```python
from build123d import *

# Parameters (mm, degrees)
SKETCH_1_W                     = 144
SKETCH_1_H                     = 144
SKETCH_1_R                     = 1.65
SKETCH_1_W_2                   = 11.212967435
SKETCH_1_H_2                   = 64.771297792
SKETCH_1_W_3                   = 88
SKETCH_1_H_3                   = 84
EXTRUDE_79X92_DEPTH            = 2
SKETCH_2_R                     = 2.75
M3_D5P5_1P1_90_DEPTH           = 1.1
M3_D5P5_1P1_90_DRAFT           = 45
M3_D5P5_1P1_90_PROFILE_2_DEPTH = 1.1
M3_D5P5_1P1_90_PROFILE_2_DRAFT = 45
M3_D5P5_1P1_90_PROFILE_3_DEPTH = 1.1
M3_D5P5_1P1_90_PROFILE_3_DRAFT = 45
M3_D5P5_1P1_90_PROFILE_4_DEPTH = 1.1
M3_D5P5_1P1_90_PROFILE_4_DRAFT = 45
CHAMFER_1_SIZE                 = 13


with BuildPart() as part:
    # 草图1 → 几何镂空托板_原装79x92孔距 (new body)
    with BuildSketch(Plane.XY):
        Rectangle(SKETCH_1_W, SKETCH_1_H)
        with Locations((-62, -62)):
            Circle(SKETCH_1_R, mode=Mode.SUBTRACT)
        with Locations((-62, 62)):
            Circle(SKETCH_1_R, mode=Mode.SUBTRACT)
        with Locations((62, -62)):
            Circle(SKETCH_1_R, mode=Mode.SUBTRACT)
        with Locations((62, 62)):
            Circle(SKETCH_1_R, mode=Mode.SUBTRACT)
        with Locations((-32.5, -46)):
            Circle(SKETCH_1_R, mode=Mode.SUBTRACT)
        with Locations((-32.5, 46)):
            Circle(SKETCH_1_R, mode=Mode.SUBTRACT)
        with Locations((46.5, -46)):
            Circle(SKETCH_1_R, mode=Mode.SUBTRACT)
        with Locations((46.5, 46)):
            Circle(SKETCH_1_R, mode=Mode.SUBTRACT)
        Polygon((-26, 67), (-6, 67), (-6, 55), (-41, 55), align=None, mode=Mode.SUBTRACT)
        Polygon((4.990317383, -65.990169234), (5.172518716, -53.991552536), (40.168484086, -54.52297309), (24.98801188, -66.293838123), align=None, mode=Mode.SUBTRACT)
        Polygon((-7.008299316, -65.807967901), (-6.826097982, -53.809351203), (-41.822063353, -53.277930648), (-27.005993813, -65.504299013), align=None, mode=Mode.SUBTRACT)
        with Locations((61.393516283, 0)):
            Rectangle(SKETCH_1_W_2, SKETCH_1_H_2, mode=Mode.SUBTRACT)
        with Locations((-61.393516283, 0)):
            Rectangle(SKETCH_1_W_2, SKETCH_1_H_2, mode=Mode.SUBTRACT)
        Rectangle(SKETCH_1_W_3, SKETCH_1_H_3, mode=Mode.SUBTRACT)
        Polygon((6, 55), (41, 55), (26, 67), (6, 67), align=None, mode=Mode.SUBTRACT)
    extrude(amount=EXTRUDE_79X92_DEPTH)


with BuildPart() as m3_d5p5_1p1_90_tool:
    # 草图2 → M3沉头四孔_D5p5_深1p1_90度 (with draft: the straight prism first)
    with BuildSketch(Plane.XY):
        with Locations((-32.5, -46)):
            Circle(SKETCH_2_R)
    extrude(amount=M3_D5P5_1P1_90_DEPTH)
    # M3沉头四孔_D5p5_深1p1_90度: the draft: its side faces are tilted about the plane it starts from
    m3_d5p5_1p1_90_sides = [m3_d5p5_1p1_90_tool.faces().sort_by_distance(p)[0] for p in [
        (-35.25, -46, 0.55),
    ]]
    draft(m3_d5p5_1p1_90_sides, Plane.XY, M3_D5P5_1P1_90_DRAFT)


with BuildPart() as part_1:
    add(part.part)

    # M3沉头四孔_D5p5_深1p1_90度: cut by m3_d5p5_1p1_90_tool
    add(m3_d5p5_1p1_90_tool.part, mode=Mode.SUBTRACT)


with BuildPart() as m3_d5p5_1p1_90_profile_2_tool:
    # 草图2 → M3沉头四孔_D5p5_深1p1_90度 profile 2 (with draft: the straight prism first)
    with BuildSketch(Plane.XY):
        with Locations((-32.5, 46)):
            Circle(SKETCH_2_R)
    extrude(amount=M3_D5P5_1P1_90_PROFILE_2_DEPTH)
    # M3沉头四孔_D5p5_深1p1_90度 profile 2: the draft: its side faces are tilted about the plane it starts from
    m3_d5p5_1p1_90_profile_2_sides = [m3_d5p5_1p1_90_profile_2_tool.faces().sort_by_distance(p)[0] for p in [
        (-35.25, 46, 0.55),
    ]]
    draft(m3_d5p5_1p1_90_profile_2_sides, Plane.XY, M3_D5P5_1P1_90_PROFILE_2_DRAFT)


with BuildPart() as part_2:
    add(part_1.part)

    # M3沉头四孔_D5p5_深1p1_90度 profile 2: cut by m3_d5p5_1p1_90_profile_2_tool
    add(m3_d5p5_1p1_90_profile_2_tool.part, mode=Mode.SUBTRACT)


with BuildPart() as m3_d5p5_1p1_90_profile_3_tool:
    # 草图2 → M3沉头四孔_D5p5_深1p1_90度 profile 3 (with draft: the straight prism first)
    with BuildSketch(Plane.XY):
        with Locations((46.5, -46)):
            Circle(SKETCH_2_R)
    extrude(amount=M3_D5P5_1P1_90_PROFILE_3_DEPTH)
    # M3沉头四孔_D5p5_深1p1_90度 profile 3: the draft: its side faces are tilted about the plane it starts from
    m3_d5p5_1p1_90_profile_3_sides = [m3_d5p5_1p1_90_profile_3_tool.faces().sort_by_distance(p)[0] for p in [
        (43.75, -46, 0.55),
    ]]
    draft(m3_d5p5_1p1_90_profile_3_sides, Plane.XY, M3_D5P5_1P1_90_PROFILE_3_DRAFT)


with BuildPart() as part_3:
    add(part_2.part)

    # M3沉头四孔_D5p5_深1p1_90度 profile 3: cut by m3_d5p5_1p1_90_profile_3_tool
    add(m3_d5p5_1p1_90_profile_3_tool.part, mode=Mode.SUBTRACT)


with BuildPart() as m3_d5p5_1p1_90_profile_4_tool:
    # 草图2 → M3沉头四孔_D5p5_深1p1_90度 profile 4 (with draft: the straight prism first)
    with BuildSketch(Plane.XY):
        with Locations((46.5, 46)):
            Circle(SKETCH_2_R)
    extrude(amount=M3_D5P5_1P1_90_PROFILE_4_DEPTH)
    # M3沉头四孔_D5p5_深1p1_90度 profile 4: the draft: its side faces are tilted about the plane it starts from
    m3_d5p5_1p1_90_profile_4_sides = [m3_d5p5_1p1_90_profile_4_tool.faces().sort_by_distance(p)[0] for p in [
        (43.75, 46, 0.55),
    ]]
    draft(m3_d5p5_1p1_90_profile_4_sides, Plane.XY, M3_D5P5_1P1_90_PROFILE_4_DRAFT)


with BuildPart() as part_4:
    add(part_3.part)

    # M3沉头四孔_D5p5_深1p1_90度 profile 4: cut by m3_d5p5_1p1_90_profile_4_tool
    add(m3_d5p5_1p1_90_profile_4_tool.part, mode=Mode.SUBTRACT)

    # 倒角1
    chamfer_1_edges = [part_4.edges().sort_by_distance(p)[0] for p in [
        (-72, 72, 1),
        (72, 72, 1),
        (-44, 42, 1),
        (72, -72, 1),
        (-44, -42, 1),
        (44, -42, 1),
        (44, 42, 1),
        (-72, -72, 1),
    ]]
    chamfer(chamfer_1_edges, length=CHAMFER_1_SIZE)


solid = part_4.part
```
Input: part model. Units: mm. Frame: model coordinates. A direction names the side the tool comes from. Coordinates: 2 decimals unless noted, no trailing zeros. Loops run counter-clockwise (first coordinate to the right, second up) from the corner with the lowest first, then second, coordinate; pieces in that order, holes last. Notation, with made-up numbers: (76, 67.25) - (88, 67.25) arc R15 ccw to (88, 95.25) - close; hole circle Ø8 at (64, 14). An arc over 180 degrees is marked (long way). Answer in a Markdown table with one row per item.
(1) Pin query (flat end, axial travel): P1, Ø3, axis at x = -62, y = -62, coming from the -Z side; P2, Ø4, axis at x = 47.5, y = 57.5, coming from the -Z side; P3, Ø0.6, axis at y = 63.5, z = 1, coming from the +X side. Return the tip coordinate at first contact, or that it passes through.
Model answer:
| item | result |
|---|---|
| P1 | passes through |
| P2 | stops at z = 0 |
| P3 | stops at x = 67.8 |
(2) Material intervals for L1, parallel to Y at x = 46.5, z = 1.75; L2, parallel to X at y = 19, z = 1.7; L3, parallel to Y at x = -39.5, z = 1.4, sorted ascending. Write a range as from..to.
Model answer:
| item | result |
|---|---|
| L1 | y = -72..-47.65, -44.35..44.35, 47.65..72 |
| L2 | x = -72..-67, -55.79..-44, 44..55.79, 67..72 |
| L3 | y = -72..-55.19, -53.31..-33.5, 33.5..55, 56.2..72 |
(3) Cut plane B-B on y = -3.5. Output: boundary loops of the cut face in (x, z), plus the area to 3 significant figures.
Model answer:
| item | result |
|---|---|
| outline | (-72, 0) - (-67, 0) - (-67, 2) - (-72, 2) - close; (-55.79, 0) - (-44, 0) - (-44, 2) - (-55.79, 2) - close; (44, 0) - (55.79, 0) - (55.79, 2) - (44, 2) - close; (67, 0) - (72, 0) - (72, 2) - (67, 2) - close |
| area | 67.1 mm² |
(4) Set-up query: faces 1 (the face through (66, -65, 1)), 2 (the face through (-37, 36, 1)). Return all of +Z, -Z, +X, -X, +Y, -Y with unobstructed straight access to the full face (end or side cutting, diameter ignored); none if empty.
Model answer:
| item | result |
|---|---|
| face 1 | +Z, -Z, +X, -Y |
| face 2 | +Z, -Z |
(5) Cut plane C-C on x = -62. Output: boundary loops of the cut face in (y, z), plus the area to 3 significant figures.
Model answer:
| item | result |
|---|---|
| outline | (-69, 0) - (-63.65, 0) - (-63.65, 2) - (-69, 2) - close; (-60.35, 0) - (-32.39, 0) - (-32.39, 2) - (-60.35, 2) - close; (32.39, 0) - (60.35, 0) - (60.35, 2) - (32.39, 2) - close; (63.65, 0) - (69, 0) - (69, 2) - (63.65, 2) - close |
| area | 133 mm² |
(6) Mould query, pull axis Y, two halves, no side actions, for faces 3 (the face through (37, 36, 1)), 4 (the face through (45.284, 47.115, 1.544)), 5 (the face through (-65, 66, 1)), 6 (the face through (-65, -66, 1)). Classes: pulls with the +Y half, pulls with the -Y half, needs draft (parallel to the pull), parting line crosses it, or undercut.
Model answer:
| item | result |
|---|---|
| face 3 | undercut |
| face 4 | undercut |
| face 5 | pulls with the +Y half |
| face 6 | pulls with the -Y half |
(7) Cut plane A-A on x = 46.5. Output: boundary loops of the cut face in (y, z).
Model answer:
| item | result |
|---|---|
| outline | (-72, 0) - (-48.75, 0) - (-47.65, 1.1) - (-47.65, 2) - (-72, 2) - close; (-44.35, 1.1) - (-43.25, 0) - (43.25, 0) - (44.35, 1.1) - (44.35, 2) - (-44.35, 2) - close; (47.65, 1.1) - (48.75, 0) - (72, 0) - (72, 2) - (47.65, 2) - close |
(8) Cut plane D-D on y = 62. Output: boundary loops of the cut face in (x, z).
Model answer:
| item | result |
|---|---|
| outline | (-69, 0) - (-63.65, 0) - (-63.65, 2) - (-69, 2) - close; (-60.35, 0) - (-32.25, 0) - (-32.25, 2) - (-60.35, 2) - close; (-6, 0) - (6, 0) - (6, 2) - (-6, 2) - close; (32.25, 0) - (60.35, 0) - (60.35, 2) - (32.25, 2) - close; (63.65, 0) - (69, 0) - (69, 2) - (63.65, 2) - close |
